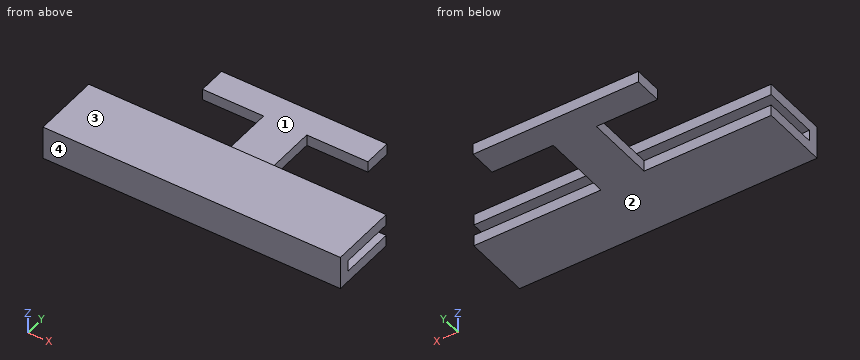
```python
from build123d import *

# Parameters (mm, degrees)
SKETCH1_W           = 80
SKETCH1_H           = 15
BOSS_EXTRUDE1_DEPTH = 3
BOSS_EXTRUDE2_DEPTH = 3
SKETCH2_W           = 80
SKETCH2_H           = 3
BOSS_EXTRUDE3_DEPTH = 3


with BuildPart() as part:
    # Sketch1 → Boss-Extrude1 (new body)
    with BuildSketch(Plane.XY):
        Rectangle(SKETCH1_W, SKETCH1_H)
    extrude(amount=BOSS_EXTRUDE1_DEPTH)



with BuildPart() as body_2:
    # Sketch3 → Boss-Extrude2 (new body)
    with BuildSketch(Plane(origin=(0, 0, -3), x_dir=(-1, 0, 0), z_dir=(0, 0, -1))):
        Polygon((40, -7.5), (-40, -7.5), (-40, 7.5), (-5.8, 7.5), (-5.8, 26.25), (-22.25, 26.25), (-22.25, 33.75), (22.25, 33.75), (22.25, 26.25), (5.8, 26.25), (5.8, 7.5), (40, 7.5), align=None)
    extrude(amount=BOSS_EXTRUDE2_DEPTH)


with BuildPart() as part_1:
    add(part.part)

    add(body_2.part)  # Boss-Extrude3 merges body 2
    # Sketch2 → Boss-Extrude3 (add)
    with BuildSketch(Plane(origin=(0, -7.5, 0), x_dir=(1, 0, 0), z_dir=(0, 1, 0))):
        with Locations((0, 4.5)):
            Rectangle(SKETCH2_W, SKETCH2_H)
        with Locations((0, 1.5)):
            Rectangle(SKETCH2_W, SKETCH2_H)
        with Locations((0, -1.5)):
            Rectangle(SKETCH2_W, SKETCH2_H)
    extrude(amount=-BOSS_EXTRUDE3_DEPTH)


solid = part_1.part
```
For this review, take the finished solid that the model builds, in its own axes (mm). Face numbers are marked on the shaded views. Give positions to 0.01 mm unless a question says otherwise; leave off trailing zeros. Write each loop counter-clockwise with the first axis right and the second up, starting at its lowest first coordinate (ties: lowest second). Pieces come first, ordered by that corner, then holes. Notation, with made-up numbers: M 23,67.5 L 30,67.5 A18 cw 30,86.5 Z; hole C 66.5,-29.5 d8. An arc over 180 degrees is marked long. One line per item, written item: value.
1) The part is to be moulded in two halves that separate along Z. For the marked faces 1, 2, 3 and 4, say which applies: +Z half, -Z half, draft (parallel to the pull), parting line (faces both ways), or undercut.
Results are:
face 1: undercut
face 2: -Z half
face 3: +Z half
face 4: draft
2) Take a section at C-C, the plane z = 0.75. Write out the cut boundary in (x, y).
Results are:
outline: M -40,-10.5 L 40,-10.5 L 40,7.5 L -40,7.5 Z
3) Take a section at B-B, the plane x = -20. Write out the cut boundary in (y, z).
Results are:
outline: M -10.5,-6 L 7.5,-6 L 7.5,-3 L -7.5,-3 L -7.5,0 L 7.5,0 L 7.5,3 L -10.5,3 Z; M 26.25,-6 L 33.75,-6 L 33.75,-3 L 26.25,-3 Z
4) Take a section at A-A, the plane y = 6.5. Write out the cut boundary in (x, z).
Results are:
outline: M -40,-6 L 40,-6 L 40,-3 L -40,-3 Z; M -40,0 L 40,0 L 40,3 L -40,3 Z
5) For line 1 (Y direction, x = 16, z = -4.5); line 2 (Z direction, x = -36, y = -5.5); line 3 (Y direction, x = 32.5, z = -1.25), list the stretches that pass through material, from the lowest coordinate up. Write a range as from..to.
Results are:
line 1: y = -10.5..7.5, 26.25..33.75
line 2: z = -6..-3, 0..3
line 3: y = -10.5..-7.5
6) Take a section at D-D, the plane y = 23.5. Write out the cut boundary in (x, z).
Results are:
outline: M -5.8,-6 L 5.8,-6 L 5.8,-3 L -5.8,-3 Z
7) For P1, Ø3.5, axis at y = 17, z = -4.5, coming from the -X side; P2, Ø3, axis at y = 19.5, z = -3, coming from the +X side; P3, Ø3.5, axis at x = 7.5, z = 1.5, coming from the +Y side; P4, Ø12.5, axis at x = 16.5, y = 17, coming from the +Z side, all flat-tipped, find the tip position at first contact; note any pin that passes through.
Results are:
P1: stops at x = -5.8
P2: stops at x = 5.8
P3: stops at y = 7.5
P4: passes through
